from build123d import *

# Parameters (mm, degrees)
BASE_FLANGE1_DEPTH                     = 577.85
SKETCH5_W                              = 369.801004036
SKETCH5_H                              = 271.212830699
CE_00_NOTCH_DEPTH                      = 254
SKETCH9_R                              = 3.175
CE_00_HOLES_0_250_SIDE_9_PLACES_DEPTH  = 7.62
SKETCH10_R                             = 3.175
CE_00_HOLES_0_250_ANGLE_2_PLACES_DEPTH = 7.62
SKETCH8_R                              = 3.175
CE_00_HOLES_0_250_TOP_3_PLACES_DEPTH   = 7.62
FILLET1_R                              = 4.7752


# Sheet-metal steps are written as plain solids
with BuildPart() as part:
    # Sketch1 → Base-Flange1 (new body)
    with BuildSketch(Plane.XY):
        with BuildLine():
            Line((144.4752, -233.3752), (144.4752, 65.007753898))
            ThreePointArc((144.4752, 65.007753898), (144.388194306, 65.445161061), (144.140423051, 65.815976949))
            Line((144.140423051, 65.815976949), (65.815976949, 144.140423051))
            ThreePointArc((65.815976949, 144.140423051), (65.445161061, 144.388194306), (65.007753898, 144.4752))
            Line((65.007753898, 144.4752), (-60.325, 144.4752))
            Line((-60.325, 144.4752), (-60.325, 146.7612))
            Line((-60.325, 146.7612), (65.007753898, 146.7612))
            ThreePointArc((65.007753898, 146.7612), (66.319975388, 146.500182917), (67.432423051, 145.756869153))
            Line((67.432423051, 145.756869153), (145.756869153, 67.432423051))
            ThreePointArc((145.756869153, 67.432423051), (146.500182917, 66.319975388), (146.7612, 65.007753898))
            Line((146.7612, 65.007753898), (146.7612, -233.3752))
            Line((146.7612, -233.3752), (144.4752, -233.3752))
        make_face()
    extrude(amount=-BASE_FLANGE1_DEPTH)

    # Sketch5 → CE-00 Notch (cut, symmetric)
    with BuildSketch(Plane(origin=(0, 0, 0), x_dir=(0, 0, -1), z_dir=(1, 0, 0))):
        with Locations((534.150502018, 141.95641535)):
            Rectangle(SKETCH5_W, SKETCH5_H)
    extrude(amount=CE_00_NOTCH_DEPTH, both=True, mode=Mode.SUBTRACT)

    # Sketch9 → CE-00 Holes 0.250 Side 9 Places (cut)
    with BuildSketch(Plane(origin=(146.7612, 0, 0), x_dir=(0, 0, -1), z_dir=(1, 0, 0))):
        with Locations(Location((31.75, -217.5002, 0), (0, 0, 90))):
            Circle(SKETCH9_R)
        with Locations(Location((203.2, -217.5002, 0), (0, 0, 90))):
            Circle(SKETCH9_R)
        with Locations(Location((374.65, -217.5002, 0), (0, 0, 90))):
            Circle(SKETCH9_R)
        with Locations(Location((546.1, -217.5002, 0), (0, 0, 90))):
            Circle(SKETCH9_R)
        with Locations(Location((546.1, -11.1252, 0), (0, 0, 90))):
            Circle(SKETCH9_R)
        with Locations(Location((374.65, -11.1252, 0), (0, 0, 90))):
            Circle(SKETCH9_R)
        with Locations(Location((22.225, 11.0998, 0), (0, 0, 90))):
            Circle(SKETCH9_R)
        with Locations(Location((22.225, -103.2002, 0), (0, 0, 90))):
            Circle(SKETCH9_R)
        with Locations(Location((555.625, -114.3127, 0), (0, 0, 90))):
            Circle(SKETCH9_R)
    extrude(amount=-CE_00_HOLES_0_250_SIDE_9_PLACES_DEPTH, mode=Mode.SUBTRACT)

    # Sketch10 → CE-00 Holes 0.250 Angle 2 Places (cut)
    with BuildSketch(Plane(origin=(106.594646102, 106.594646102, 0), x_dir=(0, 0, -1), z_dir=(0.7071067811865511, 0.707106781186544, 0))):
        with Locations(Location((22.225, 3.025193073, 0), (0, 0, 90))):
            Circle(SKETCH10_R)
        with Locations(Location((327.025, 3.025193073, 0), (0, 0, 90))):
            Circle(SKETCH10_R)
    extrude(amount=-CE_00_HOLES_0_250_ANGLE_2_PLACES_DEPTH, mode=Mode.SUBTRACT)

    # Sketch8 → CE-00 Holes 0.250 Top 3 Places (cut)
    with BuildSketch(Plane(origin=(0, 146.7612, 0), x_dir=(1, 0, 0), z_dir=(0, 1, 0))):
        with Locations(Location((-38.1, 31.75, 0), (0, 0, 180))):
            Circle(SKETCH8_R)
        with Locations(Location((-38.1, 317.5, 0), (0, 0, 180))):
            Circle(SKETCH8_R)
        with Locations(Location((-38.1, 174.625, 0), (0, 0, 180))):
            Circle(SKETCH8_R)
    extrude(amount=-CE_00_HOLES_0_250_TOP_3_PLACES_DEPTH, mode=Mode.SUBTRACT)

    # Fillet1
    fillet1_edges = [part.edges().sort_by_distance(p)[0] for p in [
        (145.6182, -233.3752, 0),
        (-60.325, 145.6182, 0),
        (145.6182, -233.3752, -577.85),
        (-60.325, 145.6182, -349.25),
        (145.6182, 6.35, -577.85),
    ]]
    fillet(fillet1_edges, radius=FILLET1_R)


solid = part.part
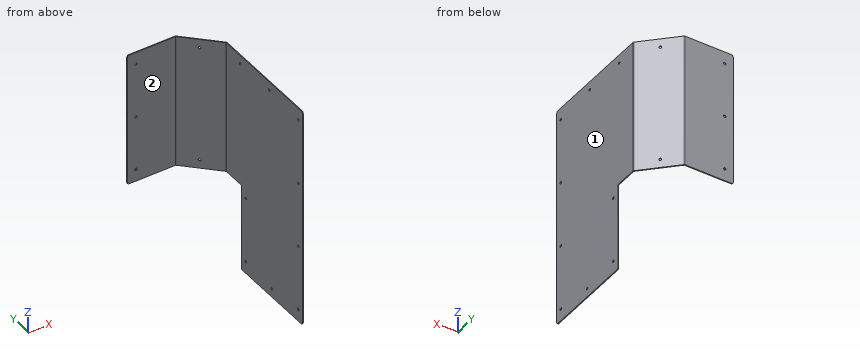
Work out the finished part from the listing and answer in its coordinate system (mm). Face numbers are marked on the shaded views. A direction names the side the tool comes from. Coordinates: 2 decimals unless noted, no trailing zeros. Loops run counter-clockwise (first coordinate to the right, second up) from the corner with the lowest first, then second, coordinate; pieces in that order, holes last. Notation, with made-up numbers: (-14, -31.75) -> (-4, -31.75) arc R13 cw to (-4, -8.75) -> close; hole circle Ø6 at (-19, 58). An arc over 180 degrees is marked (long way). Write each question's results on one line, items separated by ' | '. Start each with the question number.
1) Find section B-B on y = -191.5. Determine the outline of the cut face in (x, z).
2) For the marked faces 1 and 2, determine the directions among +Z, -Z, +X, -X, +Y, -Y from which every point of the face is accessible in a straight line to the end or side of a thin tool.
3) Find section C-C on x = 43. Determine the outline of the cut face in (y, z).
4) Flat-ended cylindrical pins translate along their axes: P1, Ø5.5, axis at x = -38.1, z = -174.625, coming from the +Y side; P2, Ø5, axis at x = -26.5, z = -118, coming from the -Y side; P3, Ø12, axis at y = 30, z = -211, coming from the -X side; P4, Ø2.5, axis at x = 146, z = -417, coming from the +Y side. Find the tip coordinate at first contact, or state that the pin passes through.
5) Consider line 1 along Y through (x, z) = (145, -374); line 2 along Y through (x, z) = (145.75, -374.65); line 3 along Y through (x, z) = (64, -217.5). Determine where each line is inside the solid, lowest interval first.
6) Find section A-A on z = -69.5. Determine the outline of the cut face in (x, y) (3 decimals).
Response values:
1) outline: (144.48, -577.85) -> (146.76, -577.85) -> (146.76, 0) -> (144.48, 0) -> close
2) face 1: +Z, -Z, +X, +Y, -Y | face 2: +Z, -Z, -X, -Y
3) outline: (144.48, -349.25) -> (146.76, -349.25) -> (146.76, 0) -> (144.48, 0) -> close
4) P1: passes through | P2: stops at y = 144.48 | P3: stops at x = 144.48 | P4: stops at y = 6.35
5) line 1: y = -233.38 to -220.61, -214.39 to -14.23, -8.02 to 6.35 | line 2: y = -233.38 to -220.68, -214.33 to -14.3, -7.95 to 6.35 | line 3: y = 144.48 to 146.76
6) outline: (-60.325, 144.475) -> (65.008, 144.475) arc R1.143 cw to (65.816, 144.14) -> (144.14, 65.816) arc R1.143 cw to (144.475, 65.008) -> (144.475, -233.375) -> (146.761, -233.375) -> (146.761, 65.008) arc R3.429 ccw to (145.757, 67.432) -> (67.432, 145.757) arc R3.429 ccw to (65.008, 146.761) -> (-60.325, 146.761) -> close
